```python
from build123d import *

# Parameters (mm, degrees)
SKETCH1_R            = 7.5
BOSS_EXTRUDE1_DEPTH  = 22
SKETCH3_R            = 7.5
BOSS_EXTRUDE2_DEPTH  = 2.54
M3_CLEARANCE_HOLE1_D = 3.4
SKETCH4_R            = 3
BOSS_EXTRUDE4_DEPTH  = 40
FILLET1_R            = 5
SKETCH12_W           = 15.000000000000002
SKETCH12_H           = 35.32384224330768
CUT_EXTRUDE1_DEPTH   = 0.4
CIRPATTERN2_COUNT    = 2
CIRPATTERN2_ANGLE    = 90.0000000000002


with BuildPart() as part:
    # Sketch1 → Boss-Extrude1 (new body)
    with BuildSketch(Plane(origin=(0, 0, 0), x_dir=(1, 0, 0), z_dir=(0, 1, 0))):
        with Locations(Location((0, 0, 0), (0, 0, 270))):
            Circle(SKETCH1_R)
        with BuildLine():
            Line((-1.5199999999999996, 3.705350860579872), (-1.52, 5.24))
            Line((-1.52, 5.24), (1.52, 5.24))
            Line((1.52, 5.24), (1.5199999999999996, 3.705350860579872))
            ThreePointArc((1.5199999999999994, 3.7053508605798724), (3.3262309751428867, 2.2307425893634614), (4.005, 0))
            ThreePointArc((4.005, -9.8e-16), (-2.2307425893634596, -3.326230975142888), (-1.5199999999999998, 3.7053508605798724))
        make_face(mode=Mode.SUBTRACT)
    extrude(amount=BOSS_EXTRUDE1_DEPTH)

    # Sketch3 → Boss-Extrude2 (add)
    with BuildSketch(Plane(origin=(0, 22, 0), x_dir=(1, 0, 0), z_dir=(0, 1, 0))):
        with Locations(Location((0, 0, 0), (0, 0, 270))):
            Circle(SKETCH3_R)
    extrude(amount=BOSS_EXTRUDE2_DEPTH)

    # M3 Clearance Hole1 (through all)
    with Locations(Plane(origin=(0, 24.54, 0), x_dir=(1, 0, 0), z_dir=(0, 1, 0))):
        with Locations((0, 0)):
            Hole(M3_CLEARANCE_HOLE1_D / 2)

    # Sketch4 → Boss-Extrude4 (add)
    with BuildSketch(Plane(origin=(0, 24.54, 0), x_dir=(1, 0, 0), z_dir=(0, 1, 0))):
        with Locations(Location((0, 0, 0), (0, 0, 270))):
            Circle(SKETCH4_R)
    extrude(amount=BOSS_EXTRUDE4_DEPTH)

    # Fillet1
    # the kernel refuses this fillet: 5 mm, written as the material it adds along each edge
    with BuildSketch(Plane(origin=(0, 24.54, 0), x_dir=(-1.8e-16, 0, 1), z_dir=(-1, 0, -1.8e-16))) as fillet1_piece_1:
        with BuildLine():
            CenterArc((8, 4.974937185533101), FILLET1_R, 180, 84.26082952273322)
            Line((3, 4.974937185533101), (2.9, 4.974937185533101))
            Line((2.9, 4.974937185533101), (2.9, 0))
            Line((2.9, 0), (3, -0.10000000000000142))
            ThreePointArc((3, -0.10000000000000142), (5.25, -0.10000000000000142), (7.49, -0.09949874371066159))
            Line((7.49, -0.09949874371066159), (7.5, 0))
        make_face()
    revolve(axis=Axis((0, 24.54, 0), (0, 1, 0)))

    # Sketch12 → Cut-Extrude1 (cut)
    with BuildSketch(Plane.ZY.offset(3.0000000000000004)):
        with Locations((0, 47.17685830718694)):
            Rectangle(SKETCH12_W, SKETCH12_H)
    cut_extrude1 = extrude(amount=-CUT_EXTRUDE1_DEPTH, mode=Mode.SUBTRACT)

    # CirPattern2: Cut-Extrude1 ×2 about axis
    cirpattern2_axis = Axis((0, 64.54, 0), (0, 1, 0))
    for i in range(1, CIRPATTERN2_COUNT):
        add(cut_extrude1.rotate(cirpattern2_axis, i * CIRPATTERN2_ANGLE / (CIRPATTERN2_COUNT - 1)), mode=Mode.SUBTRACT)


solid = part.part
```
Verification items for the finished model (mm, model axes). A direction names the side the tool comes from. Round coordinates to 2 decimals unless told otherwise and drop trailing zeros. Write each loop counter-clockwise with the first axis right and the second up, starting at its lowest first coordinate (ties: lowest second). Pieces come first, ordered by that corner, then holes.
1. Gauge pin test, flat ends, axial feed: P1, Ø1.2, axis at y = 13.5, z = -4.5, coming from the +X side; P2, Ø3, axis at x = -3, y = 17.5, coming from the -Z side; P3, Ø1.7, axis at y = 6.5, z = -4.5, coming from the -X side. Record the tip position at first contact, or that the pin passes through.
2. Section check D-D on y = 47.5. Enter the section's corners in (x, z).
3. Access from +Z, -Z, +X, -X, +Y, -Y to the whole of each face (thin tool, end or side, straight path). Record for faces 5 (the flat face through (1.52, 11, -4)), 6 (the flat face through (0, 47, 2.6)), 7 (the cylindrical face through (2.175, 46.782, -2.066)), 8 (the cylindrical face through (0.33, 12.098, -7.493)), 9 (the flat face through (-2.6, 47, 0)).
4. Section check A-A on z = 0. Enter the section's corners in (x, y) (3 decimals), plus the area to 3 significant figures.
5. Draft check along Z on faces 1 (the flat face through (0, 11, -5.24)), 2 (the cylindrical face through (-2.13, 46.78, 2.11)), 3 (the flat face through (0, 64.54, 0)), 4 (the flat face through (0, 22, -2)). Enter one of: +Z half, -Z half, draft (parallel to the pull), parting line (faces both ways), or undercut.
6. Section check B-B on y = 15. Enter the section's corners in (x, z) (3 decimals), plus the area to 3 significant figures.
7. Scan lines: L1, parallel to Y at x = -1.5, z = -2; L2, parallel to X at y = 6, z = -2.5; L3, parallel to X at y = 35, z = -1.5. Record each from-to range of solid material in increasing order.
8. Section check C-C on x = 0. Enter the section's corners in (y, z) (3 decimals), plus the area to 3 significant figures.
Answer:
1. P1: stops at x = 6.41
1. P2: stops at z = -7.35
1. P3: stops at x = -6.55
2. outline: (-2.6, -1.5) arc R3 ccw (long way) to (1.5, 2.6) - (-1.5, 2.6) arc R3 ccw to (-2.6, 1.5) - close
3. face 5: -Y
3. face 6: +Z, +X, -X, +Y
3. face 7: +Y
3. face 8: +Y, -Y
3. face 9: +Z, -Z, -X, +Y
4. outline: (-7.5, 0) - (-4.005, 0) - (-4.005, 22) - (-1.7, 22) - (-1.7, 24.54) - (1.7, 24.54) - (1.7, 22) - (4.005, 22) - (4.005, 0) - (7.5, 0) - (7.5, 24.54) arc R5 cw to (3, 29.515) - (3, 64.54) - (-2.6, 64.54) - (-2.6, 29.515) - (-3, 29.515) arc R5 cw to (-7.5, 24.54) - close
4. area: 420 mm2
5. face 1: undercut
5. face 2: +Z half
5. face 3: draft
5. face 4: undercut
6. outline: circle Ø15 at (0, 0); hole (-1.52, -5.24) - (1.52, -5.24) - (1.52, -3.705) arc R4.005 ccw (long way) to (-1.52, -3.705) - close
6. area: 122 mm2
7. L1: y = 22 to 64.54
7. L2: x = -7.07 to -3.13, 3.13 to 7.07
7. L3: x = -2.6 to 2.6
8. outline: (0, -7.5) - (24.54, -7.5) arc R5 cw to (29.515, -3) - (64.54, -3) - (64.54, 2.6) - (29.515, 2.6) - (29.515, 3) arc R5 cw to (24.54, 7.5) - (0, 7.5) - (0, 4.005) - (22, 4.005) - (22, 1.7) - (24.54, 1.7) - (24.54, -1.7) - (22, -1.7) - (22, -5.24) - (0, -5.24) - close
8. area: 393 mm2
